from build123d import *

# Parameters (mm, degrees)
SKETCH_1_W          = 220
SKETCH_1_H          = 120
EXTRUDE_1_DEPTH     = 10
CUT_EXTRUDE_1_DEPTH = 10
SKETCH_5_W          = 44.73
SKETCH_5_H          = 14.54
EXTRUDE_2_DEPTH     = 15


with BuildPart() as part:
    # 草图1 → 凸台-拉伸1 (new body)
    with BuildSketch(Plane.XY):
        with Locations((110, 60)):
            Rectangle(SKETCH_1_W, SKETCH_1_H)
    extrude(amount=EXTRUDE_1_DEPTH)

    # 草图2 → 切除-拉伸1 (cut)
    with BuildSketch(Plane.XY.offset(10)):
        Polygon((220, 120), (30, 120), (30, 80), (190, 80), (190, 115), (220, 115), align=None)
        Polygon((220, 0), (220, 5), (190, 5), (190, 40), (30, 40), (30, 0), align=None)
    extrude(amount=-CUT_EXTRUDE_1_DEPTH, mode=Mode.SUBTRACT)

    # 草图5 → 凸台-拉伸2 (add)
    with BuildSketch(Plane(origin=(220, 0, 0), x_dir=(0, 0, -1), z_dir=(1, 0, 0))):
        with Locations((-5, 60)):
            Rectangle(SKETCH_5_W, SKETCH_5_H)
    extrude_2 = extrude(amount=-EXTRUDE_2_DEPTH)

    # 镜向1: 凸台-拉伸2 across plane
    add(extrude_2.mirror(Plane(origin=(110, 0, 0), x_dir=(0, 0, 1), z_dir=(1, 0, 0))))


solid = part.part
Could you check a few things on this model? Use its own coordinates, in mm. A direction names the side the tool comes from. Give positions to 0.01 mm unless a question says otherwise; leave off trailing zeros. Order: outer loops, then holes, each group sorted by start corner. A loop starts at its lowest first (then second) coordinate and runs counter-clockwise, first axis right, second up.
Item 1: If we section it at A-A, the plane z = 15: Write out the boundary of the cut face in (x, y), plus the area to 3 significant figures.
Item 2: If we section it at C-C, the plane y = 63.5: Write out the boundary of the cut face in (x, z) (3 decimals).
Item 3: If we mould it in two halves opening along X, with no side actions, what happens to faces 6 (the face through (213, 67.27, 19)), 7 (the face through (205, 60, 19))? For each: pulls with the +X half, pulls with the -X half, needs draft (parallel to the pull), parting line crosses it, or undercut.
Item 4: For faces 1 (the face through (15, 60, 19)), 2 (the face through (7, 52.73, -9)), 3 (the face through (109, 80, 5)), 4 (the face through (213, 52.73, 19)), 5 (the face through (7, 67.27, -9)), which set-ups out of +Z, -Z, +X, -X, +Y, -Y let a thin tool reach every point of the face, with its end or its side?
Item 5: If we section it at D-D, the plane x = 40.5: Write out the boundary of the cut face in (y, z), plus the area to 3 significant figures.
Item 6: I need wall thicknesses on line 1 (X direction, y = 35.5, z = 1); line 2 (X direction, y = 67, z = -14); line 3 (Z direction, x = 124.5, y = 40.5). Which ranges of each line are inside material? Lowest first, please.
Item 7: If we section it at B-B, the plane y = 18: Write out the boundary of the cut face in (x, z), plus the area to 3 significant figures.
Item 8: I'm going to push flat-ended pins straight in: pin 1 (16.5 mm diameter, centred on x = 214, z = 19.5, fed in from +Y); pin 2 (1 mm diameter, centred on x = 78, y = 44.5, fed in from +Z); pin 3 (7.5 mm diameter, centred on x = 6.5, z = -6.5, fed in from -Y). Where does each tip first touch, or does it pass through?
Values:
1. outline: (0, 52.73) - (15, 52.73) - (15, 67.27) - (0, 67.27) - close; (205, 52.73) - (220, 52.73) - (220, 67.27) - (205, 67.27) - close
1. area: 436 mm2
2. outline: (0, -17.365) - (15, -17.365) - (15, 0) - (205, 0) - (205, -17.365) - (220, -17.365) - (220, 27.365) - (205, 27.365) - (205, 10) - (15, 10) - (15, 27.365) - (0, 27.365) - close
3. face 6: needs draft
3. face 7: undercut
4. face 1: +Z, +Y, -Y
4. face 2: -Z, +X, -X, -Y
4. face 3: +Z, -Z, +Y
4. face 4: +Z, +X, -X, -Y
4. face 5: -Z, +X, -X, +Y
5. outline: (40, 0) - (80, 0) - (80, 10) - (40, 10) - close
5. area: 400 mm2
6. line 1: x = 0 to 30, 190 to 220
6. line 2: x = 0 to 15, 205 to 220
6. line 3: z = 0 to 10
7. outline: (0, 0) - (30, 0) - (30, 10) - (0, 10) - close; (190, 0) - (220, 0) - (220, 10) - (190, 10) - close
7. area: 600 mm2
8. pin 1: stops at y = 67.27
8. pin 2: stops at z = 10
8. pin 3: stops at y = 52.73
